from build123d import *

# Parameters (mm, degrees)
CUT_EXTRUDE1_DEPTH = 1
FILLET1_R          = 0.2


with BuildPart() as part:
    # Sketch1 → Revolve1 (revolve)
    with BuildSketch(Plane(origin=(0, 0, 0), x_dir=(1, 0, 0), z_dir=(0, 1, 0))):
        with BuildLine():
            Line((0, 0), (25.5, 0))
            Line((25.5, 0), (25.5, 0.95))
            Line((25.5, 0.95), (1.25, 0.95))
            Line((1.25, 0.95), (1.25, 1.6))
            ThreePointArc((1.25, 1.6), (0.349547808, 1.015197025), (0, 0))
        make_face()
    revolve(axis=Axis((0, 0, 0), (1, 0, 0)))

    # Sketch2 → Cut-Extrude1 (cut)
    with BuildSketch(Plane(origin=(0, 0, 0), x_dir=(0, 0, -1), z_dir=(1, 0, 0))):
        with BuildLine():
            Line((0.375, -1.925921717), (-0.375, -1.925921717))
            Line((-0.375, -1.925921717), (-0.375, -0.649519053))
            ThreePointArc((-0.375, -0.649519053), (-0.75, 0), (-0.375, 0.649519053))
            Line((-0.375, 0.649519053), (-0.375, 1.925921717))
            Line((-0.375, 1.925921717), (0.375, 1.925921717))
            Line((0.375, 1.925921717), (0.375, 0.649519053))
            ThreePointArc((0.375, 0.649519053), (0.75, 0), (0.375, -0.649519053))
            Line((0.375, -0.649519053), (0.375, -1.925921717))
        make_face()
    extrude(amount=CUT_EXTRUDE1_DEPTH, mode=Mode.SUBTRACT)

    # Fillet1
    # the kernel refuses this fillet: 0.2 mm, written as the material it takes off along each edge
    with BuildSketch(Plane(origin=(25.5, 0, 0), x_dir=(0, 0, -1), z_dir=(0, -1, 0))) as fillet1_piece_1:
        with BuildLine():
            CenterArc((0.95 - FILLET1_R, -FILLET1_R), FILLET1_R, 0, 90)
            Line((0.95, -FILLET1_R), (0.95, 0))
            Line((0.95, 0), (0.95 - FILLET1_R, 0))
        make_face()
    revolve(axis=Axis((25.5, 0, 0), (1, 0, 0)), mode=Mode.SUBTRACT)
    with BuildSketch(Plane(origin=(1.25, 0, 0), x_dir=(0, 0, -1), z_dir=(0, -1, 0))) as fillet1_piece_2:
        with BuildLine():
            CenterArc((1.3193938, -0.2), FILLET1_R, 335.582123666, 114.417876334)
            ThreePointArc((1.501504746, -0.282677709), (1.557180013, -0.143578479), (1.6, 0))
            Line((1.6, 0), (1.3193938, 0))
        make_face()
    revolve(axis=Axis((1.25, 0, 0), (1, 0, 0)), mode=Mode.SUBTRACT)


solid = part.part
Geometry check sheet. Reference: the model listing, model coordinates, mm. A direction names the side the tool comes from. Round coordinates to 2 decimals unless told otherwise and drop trailing zeros. Loops run counter-clockwise (first coordinate to the right, second up) from the corner with the lowest first, then second, coordinate; pieces in that order, holes last.
Item 1: Cross-section at A-A on z = 0. Record the boundary of the cut face in (x, y), then the cut area to 3 significant figures.
Item 2: Cross-section at C-C on x = 23.75. Record the boundary of the cut face in (y, z), then the cut area to 3 significant figures.
Item 3: Mould release check, pull along Y, two halves, no side actions. Record for faces 1 (the flat face through (25.5, 0, 0)), 2 (the cylindrical face through (0.58, -0.01, 0.75)), 3 (the cylindrical face through (13.11, 0.04, 0.95)): pulls with the +Y half, pulls with the -Y half, needs draft (parallel to the pull), parting line crosses it, or undercut.
Item 4: Access from +Z, -Z, +X, -X, +Y, -Y to the whole of each face (thin tool, end or side, straight path). Record for faces 4 (the flat face through (0.7, -1, -0.375)), 5 (the flat face through (1, 0, 0)).
Item 5: Thickness scan on line 1 (X direction, y = -0.65, z = -0.1); line 2 (Z direction, x = 9, y = 0.1); line 3 (Y direction, x = 2.25, z = 0.05). Record the ranges inside material, lowest first.
Item 6: Gauge pin test, flat ends, axial feed: pin 1 (0.9 mm diameter, centred on x = 1, y = 1, fed in from -Z); pin 2 (0.8 mm diameter, centred on y = 0, z = 0, fed in from -X). Record the tip position at first contact, or that the pin passes through.
Item 7: Cross-section at B-B on y = 0. Record the boundary of the cut face in (x, z), then the cut area to 3 significant figures.
Answer sheet:
1. outline: (1, -1.51) arc R0.2 ccw to (1.25, -1.32) - (1.25, -0.95) - (25.3, -0.95) arc R0.2 ccw to (25.5, -0.75) - (25.5, 0.75) arc R0.2 ccw to (25.3, 0.95) - (1.25, 0.95) - (1.25, 1.32) arc R0.2 ccw to (1, 1.51) - close
1. area: 46.8 mm2
2. outline: circle Ø1.9 at (0, 0)
2. area: 2.84 mm2
3. face 1: needs draft
3. face 2: undercut
3. face 3: parting line crosses it
4. face 4: -X, +Y, -Y
4. face 5: -X
5. line 1: x = 1 to 25.5
5. line 2: z = -0.94 to 0.94
5. line 3: y = -0.95 to 0.95
6. pin 1: stops at z = -1.42
6. pin 2: stops at x = 1
7. outline: (0.18, -0.75) arc R1.65 ccw to (0.97, -1.5) arc R0.2 ccw to (1.25, -1.32) - (1.25, -0.95) - (25.3, -0.95) arc R0.2 ccw to (25.5, -0.75) - (25.5, 0.75) arc R0.2 ccw to (25.3, 0.95) - (1.25, 0.95) - (1.25, 1.32) arc R0.2 ccw to (0.97, 1.5) arc R1.65 ccw to (0.18, 0.75) - (1, 0.75) - (1, -0.75) - close
7. area: 47.6 mm2
